Drawing for the job (mm, zero at the part's lowest x, y, z). Coordinates: 2 decimals unless noted, no trailing zeros. Order: outer loops, then holes, each group sorted by start corner. A loop starts at its lowest first (then second) coordinate and runs counter-clockwise, first axis right, second up. Notation, with made-up numbers: M 86.5,25.5 L 109.5,25.5 A16 cw 109.5,40.5 Z; hole C -13.75,-26 d5. An arc over 180 degrees is marked long. Write item = value, one per line. Start each with the question number.
Q1. Drill centre lines: probe 1 along Y at (x, z) = (90, 0.95); probe 2 along X at (y, z) = (170, 1.6); probe 3 along Y at (x, z) = (9.5, 1). Where is each one in solid material? Low to high.
Q2. Pin check, flat tips, straight feed: P1, Ø13, axis at x = 90, y = 50, coming from the -Z side; P2, Ø3, axis at x = 10, y = 10, coming from the +Z side. Stop position of each tip, or through.
Q3. Band-saw the part on B-B on z = 1.9. State how many separate pieces and enclosed holes the cut face has, plus the area to 3 significant figures.
Q4. Band-saw the part on D-D on y = 50. Write the cut outline in (x, z).
Q5. Band-saw the part on C-C on y = 170. Write the cut outline in (x, z).
Q6. Band-saw the part on A-A on x = 90. Write the cut outline in (y, z), plus the area to 3 significant figures.
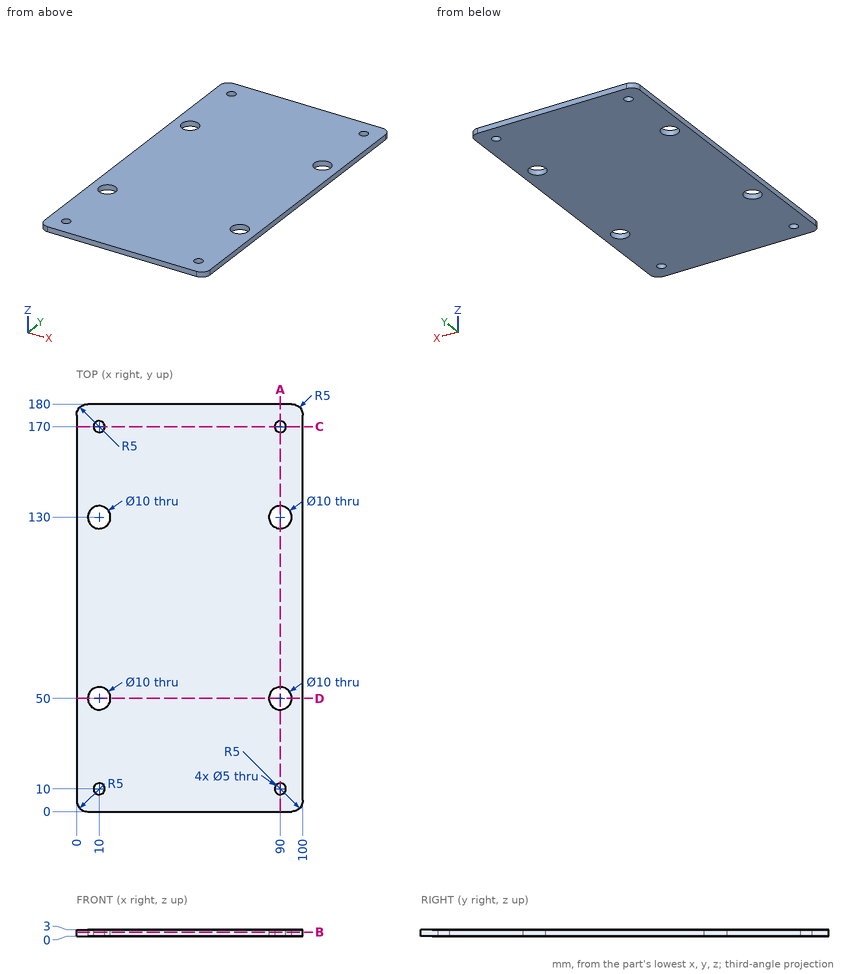
Recorded:
q1.probe_1 = 0 to 7.5, 12.5 to 45, 55 to 125, 135 to 167.5, 172.5 to 180
q1.probe_2 = 0 to 7.5, 12.5 to 87.5, 92.5 to 100
q1.probe_3 = 0 to 7.55, 12.45 to 45.03, 54.97 to 125.03, 134.97 to 167.55, 172.45 to 180
q2.P1 = 0
q2.P2 = through
q3.separate_pieces = 1
q3.enclosed_holes = 8
q3.area = 17,600 mm2
q4.outline = M 0,0 L 5,0 L 5,3 L 0,3 Z; M 15,0 L 85,0 L 85,3 L 15,3 Z; M 95,0 L 100,0 L 100,3 L 95,3 Z
q5.outline = M 0,0 L 7.5,0 L 7.5,3 L 0,3 Z; M 12.5,0 L 87.5,0 L 87.5,3 L 12.5,3 Z; M 92.5,0 L 100,0 L 100,3 L 92.5,3 Z
q6.outline = M 0,0 L 7.5,0 L 7.5,3 L 0,3 Z; M 12.5,0 L 45,0 L 45,3 L 12.5,3 Z; M 55,0 L 125,0 L 125,3 L 55,3 Z; M 135,0 L 167.5,0 L 167.5,3 L 135,3 Z; M 172.5,0 L 180,0 L 180,3 L 172.5,3 Z
q6.area = 450 mm2
